Source: CAD feature listing. Evaluate the final solid. Frame: model axes, mm. A direction names the side the tool comes from. Round coordinates to 2 decimals unless told otherwise and drop trailing zeros. Order: outer loops, then holes, each group sorted by start corner. A loop starts at its lowest first (then second) coordinate and runs counter-clockwise, first axis right, second up. Notation, with made-up numbers: (43.25, 9.5) -> (53.25, 9.5) arc R19 cw to (53.25, 43.5) -> close; hole circle Ø6 at (-17.5, 22.5). An arc over 180 degrees is marked (long way). One line per item, written item: value. Start each with the question number.
1) Reachability of faces 4 (the face through (39, 0, 10)), 5 (the face through (0, 0, 5)), 6 (the face through (145, 0, 2)), 7 (the face through (58, 1.5, 7)), 8 (the face through (72, 2, 4)) from +Z, -Z, +X, -X, +Y, -Y: full face, straight path, thin tool, end or side. Return the list, or none.
2) Section A-A (z = 5.5). Return the cut outline in (x, y).
3) Section B-B (y = 0). Return the cut outline in (x, z).
4) Section C-C (x = 103.5). Return the cut outline in (y, z), and give its area (3 significant figures).
5) Section D-D (x = 79.5). Return the cut outline in (y, z), and give its area (3 significant figures).
6) Pin query (flat end, axial travel): P1, Ø1.2, axis at y = 0, z = 3, coming from the -X side; P2, Ø5, axis at x = 79.5, z = 8, coming from the +Y side; P3, Ø2, axis at x = 10, y = -2.5, coming from the -Z side; P4, Ø4, axis at y = 0.5, z = 7.5, coming from the +X side. Return the tip coordinate at first contact, or that it passes through.
7) Mould query, pull axis X, two halves, no side actions, for faces 1 (the face through (141, 0, 8)), 2 (the face through (-3, -3.5, 4.9)), 3 (the face through (60, -1.5, 7)). Classes: pulls with the +X half, pulls with the -X half, needs draft (parallel to the pull), parting line crosses it, or undercut.
8) Ray query, L1, parallel to Z at x = 64.5, y = -4.25; L2, parallel to Y at x = 89, z = 5; L3, parallel to X at y = 0, z = 3. Return the intervals inside material, ascending.
```python
from build123d import *

# Parameters (mm, degrees)
PAD_DEPTH    = 4
SKETCH001_R  = 8
PAD001_DEPTH = 10
POCKET_DEPTH = 10.001
SKETCH003_R  = 2
PAD002_DEPTH = 8
PAD003_DEPTH = 10


with BuildPart() as part:
    # Sketch → Pad (new body)
    with BuildSketch(Plane.XY):
        with BuildLine():
            ThreePointArc((0.22695, 7.99678), (-8, 0), (0.22695, -7.99678))
            Line((0.22695, -7.99678), (141.113475, -3.99839))
            ThreePointArc((141.113475, -3.99839), (145, 0), (141.113475, 3.99839))
            Line((0.22695, 7.99678), (141.113475, 3.99839))
        make_face()
    extrude(amount=PAD_DEPTH)

    # Sketch001 → Pad001 (join)
    with BuildSketch(Plane.XY):
        Circle(SKETCH001_R)
    extrude(amount=PAD001_DEPTH)

    # Sketch002 → Pocket (cut, through all)
    with BuildSketch(Plane.XY):
        Polygon((0, -2), (-8, -6), (-8, 6), (0, 2), align=None)
    extrude(amount=POCKET_DEPTH, mode=Mode.SUBTRACT)

    # Sketch003 → Pad002 (join)
    with BuildSketch(Plane.XY):
        with Locations((141, 0)):
            Circle(SKETCH003_R)
    extrude(amount=PAD002_DEPTH)

    # Sketch004 → Pad003 (join)
    with BuildSketch(Plane.XY):
        with BuildLine():
            Line((0, 1.5), (110.000009, 1.5))
            ThreePointArc((110, -1.5), (111.5, -5e-06), (110.000009, 1.5))
            Line((110, -1.5), (0, -1.5))
            Line((0, -1.5), (0, 1.5))
        make_face()
    extrude(amount=PAD003_DEPTH)


solid = part.part
```
Findings:
1. face 4: +Z, +X, -X, +Y, -Y
1. face 5: +Z, -Z, -X
1. face 6: +Z, -Z, +X
1. face 7: +Z, +Y
1. face 8: +Z
2. outline: (-6.17, -5.09) arc R8 ccw to (7.86, -1.5) -> (110, -1.5) arc R1.5 ccw to (110, 1.5) -> (7.86, 1.5) arc R8 ccw to (-6.17, 5.09) -> (0, 2) -> (0, -2) -> close; circle Ø4 at (141, 0)
3. outline: (0, 0) -> (145, 0) -> (145, 4) -> (143, 4) -> (143, 8) -> (139, 8) -> (139, 4) -> (111.5, 4) -> (111.5, 10) -> (0, 10) -> close
4. outline: (-5.07, 0) -> (5.07, 0) -> (5.07, 4) -> (1.5, 4) -> (1.5, 10) -> (-1.5, 10) -> (-1.5, 4) -> (-5.07, 4) -> close
4. area: 58.5 mm2
5. outline: (-5.75, 0) -> (5.75, 0) -> (5.75, 4) -> (1.5, 4) -> (1.5, 10) -> (-1.5, 10) -> (-1.5, 4) -> (-5.75, 4) -> close
5. area: 64.0 mm2
6. P1: x = 0
6. P2: y = 1.5
6. P3: z = 0
6. P4: x = 143
7. face 1: needs draft
7. face 2: pulls with the -X half
7. face 3: undercut
8. L1: 0 to 4
8. L2: -1.5 to 1.5
8. L3: 0 to 145
